Build history of the part. All positions in model axes, mm. Face numbers are marked on the shaded views. Give positions to 0.01 mm unless a question says otherwise; leave off trailing zeros. Order: outer loops, then holes, each group sorted by start corner. A loop starts at its lowest first (then second) coordinate and runs counter-clockwise, first axis right, second up. Notation, with made-up numbers: (79.25, 73) - (84.25, 73) arc R29 cw to (84.25, 95) - close; hole circle Ø7 at (55.5, 25.25). An arc over 180 degrees is marked (long way). Use a Markdown table: item, result.
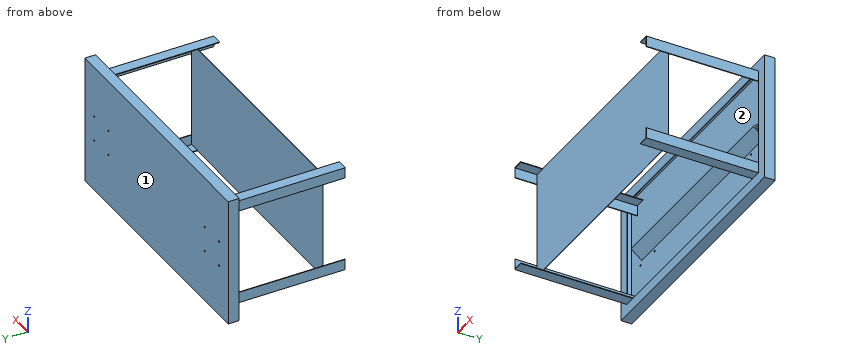
from build123d import *

# Parameters (mm, degrees)
BOSS_EXTRUDE1_DEPTH = 914.4
BOSS_EXTRUDE2_DEPTH = 457.2
BOSS_EXTRUDE3_DEPTH = 868.9975
BOSS_EXTRUDE4_START = 712.7875
SKETCH5_W           = 1676.4
SKETCH5_H           = 762
BOSS_EXTRUDE4_DEPTH = 2.657
SKETCH6_R           = 6.35
CUT_EXTRUDE1_DEPTH  = 10
BOSS_EXTRUDE5_DEPTH = 779


with BuildPart() as part:
    # Sketch1 → Boss-Extrude1 (new body, symmetric)
    with BuildSketch(Plane(origin=(0, 0, 0), x_dir=(0, 0, -1), z_dir=(1, 0, 0))):
        Polygon((-457.2, 0), (457.2, 0), (457.2, -76.2), (381, -76.2), (381, -71.4375), (452.4375, -71.4375), (452.4375, -4.7625), (-452.4375, -4.7625), (-452.4375, -71.4375), (-381, -71.4375), (-381, -76.2), (-457.2, -76.2), align=None)
    extrude(amount=BOSS_EXTRUDE1_DEPTH, both=True)

    # Sketch2 → Boss-Extrude2 (add, symmetric)
    with BuildSketch(Plane.XY):
        Polygon((-914.4, 0), (-914.4, -76.2), (-838.2, -76.2), (-838.2, -71.4375), (-909.6375, -71.4375), (-909.6375, 0), align=None)
        Polygon((909.6375, 0), (914.4, 0), (914.4, -76.2), (838.2, -76.2), (838.2, -71.4375), (909.6375, -71.4375), align=None)
    extrude(amount=BOSS_EXTRUDE2_DEPTH, both=True)

    # Sketch4 → Boss-Extrude3 (add)
    with BuildSketch(Plane.XZ.offset(4.7625)):
        Polygon((-762, 381), (-838.2, 381), (-838.2, 304.8), (-833.646, 304.8), (-833.646, 376.446), (-762, 376.446), align=None)
        Polygon((-833.646, -376.446), (-762, -376.446), (-762, -381), (-838.2, -381), (-838.2, -304.8), (-833.646, -304.8), align=None)
        Polygon((833.646, -304.8), (833.646, -376.446), (762, -376.446), (762, -381), (838.2, -381), (838.2, -304.8), align=None)
        Polygon((833.646, 376.446), (762, 376.446), (762, 381), (838.2, 381), (838.2, 304.8), (833.646, 304.8), align=None)
    extrude(amount=BOSS_EXTRUDE3_DEPTH)

    # Sketch5 → Boss-Extrude4 (add)
    with BuildSketch(Plane.XZ.offset(4.7625).offset(BOSS_EXTRUDE4_START)):
        Rectangle(SKETCH5_W, SKETCH5_H)
    extrude(amount=-BOSS_EXTRUDE4_DEPTH)

    # Sketch6 → Cut-Extrude1 (cut)
    with BuildSketch(Plane(origin=(0, 0, 0), x_dir=(1, 0, 0), z_dir=(0, 1, 0))):
        with Locations((-794.4, 90)):
            Circle(SKETCH6_R)
        with Locations((-614.4, 90)):
            Circle(SKETCH6_R)
        with Locations((-794.4, -90)):
            Circle(SKETCH6_R)
        with Locations((-614.4, -90)):
            Circle(SKETCH6_R)
        with Locations((614.4, -90)):
            Circle(SKETCH6_R)
        with Locations((794.4, -90)):
            Circle(SKETCH6_R)
        with Locations((794.4, 90)):
            Circle(SKETCH6_R)
        with Locations((614.4, 90)):
            Circle(SKETCH6_R)
    extrude(amount=-CUT_EXTRUDE1_DEPTH, mode=Mode.SUBTRACT)

    # Sketch7 → Boss-Extrude5 (add, symmetric)
    with BuildSketch(Plane(origin=(0, 0, 0), x_dir=(0, 0, -1), z_dir=(1, 0, 0))):
        Polygon((63.172612778, -4.7625), (50.8, -4.7625), (0, -66.038420526), (-50.8, -4.7625), (-63.172612778, -4.7625), (0, -80.9625), align=None)
    extrude(amount=BOSS_EXTRUDE5_DEPTH, both=True)


solid = part.part
1) Pin check, flat tips, straight feed: P1, Ø2.5, axis at y = -794.5, z = 378.5, coming from the -X side; P2, Ø5, axis at x = -836.5, y = -773, coming from the +Z side; P3, Ø2.5, axis at y = -767.5, z = 378.5, coming from the +X side. Stop position of each tip, or through.
Computed:
| item | result |
|---|---|
| P1 | stops at x = -838.2 |
| P2 | stops at z = 381 |
| P3 | stops at x = 838.2 |
2) Slice it at B-B (z = -163.5). Write the cut outline in (x, y), and give its area (3 significant figures).
Computed:
| item | result |
|---|---|
| outline | (-914.4, -76.2) - (-838.2, -76.2) - (-838.2, -71.44) - (-909.64, -71.44) - (-909.64, -4.76) - (909.64, -4.76) - (909.64, -71.44) - (838.2, -71.44) - (838.2, -76.2) - (914.4, -76.2) - (914.4, 0) - (-914.4, 0) - close; (-838.2, -717.55) - (838.2, -717.55) - (838.2, -714.89) - (-838.2, -714.89) - close |
| area | 14,500 mm² |
3) Two-plate mould, pull along X, no slides. Class the marked faces 1 and 2: +X half, -X half, draft (parallel to the pull), parting line (faces both ways), or undercut.
Computed:
| item | result |
|---|---|
| face 1 | draft |
| face 2 | undercut |
4) Slice it at A-A (x = 656). Write the cut outline in (y, z), and give its area (3 significant figures).
Computed:
| item | result |
|---|---|
| outline | (-717.55, -381) - (-714.89, -381) - (-714.89, 381) - (-717.55, 381) - close; (-80.96, 0) - (-4.76, -63.17) - (-4.76, -452.44) - (-71.44, -452.44) - (-71.44, -381) - (-76.2, -381) - (-76.2, -457.2) - (0, -457.2) - (0, 457.2) - (-76.2, 457.2) - (-76.2, 381) - (-71.44, 381) - (-71.44, 452.44) - (-4.76, 452.44) - (-4.76, 63.17) - close; hole (-66.04, 0) - (-4.76, -50.8) - (-4.76, 50.8) - close |
| area | 9,440 mm² |
5) Wall check: line 1 (Z direction, x = -614.4, y = -1.95); line 2 (X direction, y = -1.5, z = -90); line 3 (Y direction, x = 495.5, z = -104). Give the ranges that are in metal, low to high. Write a range as from..to.
Computed:
| item | result |
|---|---|
| line 1 | z = -457.2..-96.35, -83.65..83.65, 96.35..457.2 |
| line 2 | x = -914.4..-800.75, -788.05..-620.75, -608.05..608.05, 620.75..788.05, 800.75..914.4 |
| line 3 | y = -717.55..-714.89, -4.76..0 |
6) Slice it at C-C (y = -601.5). Write the cut outline in (x, z), and give its area (3 significant figures).
Computed:
| item | result |
|---|---|
| outline | (-838.2, -381) - (-762, -381) - (-762, -376.45) - (-833.65, -376.45) - (-833.65, -304.8) - (-838.2, -304.8) - close; (-838.2, 304.8) - (-833.65, 304.8) - (-833.65, 376.45) - (-762, 376.45) - (-762, 381) - (-838.2, 381) - close; (762, -381) - (838.2, -381) - (838.2, -304.8) - (833.65, -304.8) - (833.65, -376.45) - (762, -376.45) - close; (762, 376.45) - (833.65, 376.45) - (833.65, 304.8) - (838.2, 304.8) - (838.2, 381) - (762, 381) - close |
| area | 2,690 mm² |
7) Slice it at D-D (z = 399). Write the cut outline in (x, y), and give its area (3 significant figures).
Computed:
| item | result |
|---|---|
| outline | (-914.4, -76.2) - (914.4, -76.2) - (914.4, 0) - (-914.4, 0) - close; hole (-909.64, -71.44) - (909.64, -71.44) - (909.64, -4.76) - (-909.64, -4.76) - close |
| area | 18,100 mm² |
